Check sheet for the modelled part. Datum: model origin and axes. Units: mm. A direction names the side the tool comes from. Round coordinates to 2 decimals unless told otherwise and drop trailing zeros. Order: outer loops, then holes, each group sorted by start corner. A loop starts at its lowest first (then second) coordinate and runs counter-clockwise, first axis right, second up.
Autodesk Inventor part; units mm, degrees
ref_plane "YZ Plane" through (0, 0, 0) normal (1, 0, 0) x (0, 1, 0)
ref_plane "XZ Plane" through (0, 0, 0) normal (0, 1, 0) x (-1, 0, 0)
ref_plane "XY Plane" through (0, 0, 0) normal (0, 0, 1) x (1, 0, 0)
sketch "Sketch1" plane through (0, 0, 0) normal (0, 0, 1) x (1, 0, 0)
  line L0 (3, 13.65) -> (3, 2.65)
  line L1 (3, 2.65) -> (24, 2.65)
  line L2 (24, 2.65) -> (24, -9)
  line L3 (24, -9) -> (21, -9)
  line L4 (21, -9) -> (21, 0)
  line L5 (21, 0) -> (0, 0)
  line L6 (0, 0) -> (0, 13.65)
  line L7 (0, 13.65) -> (3, 13.65)
  dimension "d0" = 2.65
  dimension "d1" = 21
  dimension "d2" = 9
  dimension "d3" = 3
  dimension "d4" = 3
  dimension "d5" = 11
extrude "Extrusion1" add sketch "Sketch1" along normal blind 45
sketch "Sketch2" plane through (3, 2.65, 0) normal (1, 0, 0) x (0, 0, -1)
  line L0 (0, 11) -> (-45, 11)
  line L1 (-35, 11) -> (-28, 0)
  line L2 (-17, 0) -> (-10, 11)
  line L3 (0, 0) -> (0, 11)
  line L4 (0, 11) -> (-45, 11)
  line L5 (-45, 0) -> (-45, 11)
  line L6 (0, 0) -> (-45, 0)
  point P0 (0, -2.65)
  dimension "d10" = 10
  dimension "d11" = 10
  dimension "d38" = 11
extrude "Extrusion2" cut sketch "Sketch2" against normal through all contours L2 L6 L1 L0
ref_plane "Work Plane1" through (0, 0, 22.5) normal (0, 0, 1) x (1, 0, 0)
sketch "Sketch3" plane through (3, 2.65, 0) normal (0, 1, 0) x (1, 0, 0)
  line L0 (-3, 0) -> (18, 0)
  line L1 (6, 0) -> (9, -3)
  line L2 (9, -3) -> (12, -3)
  line L3 (12, -3) -> (15, 0)
  line L4 (6, -45) -> (9, -42)
  line L5 (9, -42) -> (12, -42)
  line L6 (12, -42) -> (15, -45)
  line L7 (21, 0) -> (0, 0)
  line L8 (0, 0) -> (0, -17)
  line L9 (0, -17) -> (-3, -17)
  line L10 (-3, -28) -> (-3, -17)
  line L11 (0, -28) -> (-3, -28)
  line L12 (0, -28) -> (0, -45)
  line L13 (21, -45) -> (0, -45)
  line L14 (21, 0) -> (21, -45)
  point P0 (10.5, -3)
  point P1 (10.5, 0)
  point P2 (10.5, -42)
  point P3 (10.5, -45)
  dimension "d14" = 45
  dimension "d15" = 45
  dimension "d16" = 3
  dimension "d17" = 3
  dimension "d18" = 3
extrude "Extrusion3" cut sketch "Sketch3" against normal through all contours L0 L3 L2 L1 | L13 L4 L5 L6
sketch "Sketch4" plane through (3, 2.65, 45) normal (1, 0, 0) x (0, 0, -1)
  line L0 (0, 0) -> (0, 11)
  line L1 (45, 0) -> (45, 11)
  line L2 (45, 11) -> (35, 11)
  line L3 (10, 11) -> (0, 11)
  point P0 (45, -2.65)
  point P1 (40.5, 5.85)
  point P2 (4.5, 5.85)
  point P3 (0, 5.5)
  point P4 (45, 5.5)
  dimension "d21" = 4.5
  dimension "d22" = 4.5
  dimension "d46" = 5.15
hole "Hole1" at (3, 8.5, 4.5) at (3, 8.5, 40.5) direction (-1, 0, 0) diameter 3.6 end through all countersink diameter 6.3 countersink angle 90
sketch "Sketch5" plane through (21, -9, 0) normal (0, -1, 0) x (1, 0, 0)
  line L0 (0, 0) -> (3, 0)
  line L1 (3, 0) -> (3, 45)
  line L2 (0, 45) -> (3, 45)
  line L3 (0, 0) -> (0, 45)
  line L4 (3, 0) -> (3, 45)
  line L5 (3, 19.1965) -> (11, 13.5983)
  line L6 (11, 13.5983) -> (11, 5.5983)
  line L7 (11, 5.5983) -> (3, 0)
  line L8 (3, 45) -> (11, 39.4017)
  line L9 (11, 39.4017) -> (11, 31.4017)
  line L10 (11, 31.4017) -> (3, 25.8035)
  line L11 (3, 0) -> (-3, 0)
  line L12 (3, 45) -> (-3, 45)
  point P0 (-21, 0)
  point P1 (3, 22.5)
  dimension "d30" = 8
  dimension "d31" = 8
  dimension "d32" = 8
  dimension "d33" = 8
  dimension "d66" = 5.5983
  dimension "d67" = 5.5983
extrude "Extrusion4" add sketch "Sketch5" against normal blind 3 contours L1 L5 L6 L7 | L8 L9 L10 L1
sketch "Sketch6" plane through (21, -6, 0) normal (0, 1, 0) x (1, 0, 0)
  line L0 (3, -19.1965) -> (11, -13.5983)
  line L1 (11, -13.5983) -> (11, -5.5983)
  line L2 (11, -5.5983) -> (3, 0)
  line L3 (3, -19.1965) -> (3, 0)
  line L4 (3, -45) -> (11, -39.4017)
  line L5 (11, -39.4017) -> (11, -31.4017)
  line L6 (11, -31.4017) -> (3, -25.8035)
  line L7 (3, -19.1965) -> (3, 0)
  line L8 (3, -45) -> (3, -25.8035)
  line L9 (3, -19.1965) -> (11, -13.5983)
  line L10 (11, -13.5983) -> (11, -5.5983)
  line L11 (11, -5.5983) -> (3, 0)
  line L12 (3, -45) -> (11, -39.4017)
  line L13 (11, -39.4017) -> (11, -31.4017)
  line L14 (11, -31.4017) -> (3, -25.8035)
  line L15 (3, -45) -> (3, -25.8035)
  point P0 (-21, 0)
  point P1 (6, -35.4017)
  point P2 (6, -9.5983)
  point P3 (7, -16.3974)
  point P4 (7, -28.6026)
  point P5 (11, -35.4017)
  point P6 (11, -9.5983)
  dimension "d62" = 3
hole "Hole2" at (27, -6, 35.4017) at (27, -6, 9.5983) direction (0, -1, 0) diameter 3.6 end through all countersink diameter 6.3 countersink angle 90
sketch "Sketch7" plane through (24, 2.65, 45) normal (0, 1, 0) x (1, 0, 0)
  circle A0 centre (-10.5, 36) radius 2
  circle A1 centre (-10.5, 9) radius 2
  circle A2 centre (-10.5, 9) radius 4
  circle A3 centre (-10.5, 36) radius 4
  line L0 (-12, 3) -> (-9, 3)
  line L1 (-24, 17) -> (-24, 28)
  line L2 (-24, 22.5) -> (-9, 22.5) construction
  point P0 (-24, 45)
  point P1 (-10.5, 3)
  dimension "d48" = 4
  dimension "d49" = 13.5
  dimension "d50" = 13.5
  dimension "d51" = 8
  dimension "d61" = 27
extrude "Extrusion5" add sketch "Sketch7" along normal blind 3
extrude "Extrusion6" cut sketch "Sketch7" against normal through all contours A0 | A1
draft "FaceDraft1" angle 30 pull direction (0, 1, 0) faces at (17.487, 4.65, 36.3219) fixed edges at (9.5, 5.65, 36)
draft "FaceDraft2" angle 30 pull direction (0, 1, 0) faces at (17.487, 4.65, 9.3219) fixed edges at (9.5, 5.65, 9)
equation "\"d30\" = d31"
equation "\"d32\" = d31"
equation "\"d33\" = d30"
equation "\"d50\" = d49"
properties part number "ESC Mount"
Item 1: Access from +Z, -Z, +X, -X, +Y, -Y to the whole of each face (thin tool, end or side, straight path). Record for faces 5 (the cylindrical face through (12.026, 2.865, 7.648)), 6 (the flat face through (16, 1, 2)), 7 (the flat face through (30, -6, 8)), 8 (the flat face through (11, 0, 22)), 9 (the flat face through (28.056, -7.521, 28.642)).
Answer:
face 5: +Y, -Y
face 6: -Z, +Y, -Y
face 7: +Z, -Z, +X, +Y
face 8: +Z, -Z, -X, -Y
face 9: +X, +Y, -Y
Item 2: Release check for a two-part mould opening along Z. For faces 1 (the flat face through (1, 13.65, 40)), 2 (the flat face through (22, -2, 0)), 3 (the flat face through (27.94, -7.52, 16.44)), 4 (the flat face through (10, 1, 44)) record: released by +Z, released by -Z, zero draft, split by the parting line, or undercut.
Answer:
face 1: zero draft
face 2: released by -Z
face 3: undercut
face 4: released by +Z
Item 3: Sectioned sample at D-D (x = 27). Record the cut outline in (y, z).
Answer:
outline: (-9, 2.1) - (-6, 2.1) - (-6, 6.45) - (-7.35, 7.8) - (-9, 7.8) - close; (-9, 11.4) - (-7.35, 11.4) - (-6, 12.75) - (-6, 17.1) - (-9, 17.1) - close; (-9, 27.9) - (-6, 27.9) - (-6, 32.25) - (-7.35, 33.6) - (-9, 33.6) - close; (-9, 37.2) - (-7.35, 37.2) - (-6, 38.55) - (-6, 42.9) - (-9, 42.9) - close
Item 4: Sectioned sample at C-C (y = 8.5). Record the cut outline in (x, z).
Answer:
outline: (0, 0) - (3, 0) - (3, 1.35) - (1.65, 2.7) - (0, 2.7) - close; (0, 6.3) - (1.65, 6.3) - (3, 7.65) - (3, 13.28) - (0, 13.28) - close; (0, 31.72) - (3, 31.72) - (3, 37.35) - (1.65, 38.7) - (0, 38.7) - close; (0, 42.3) - (1.65, 42.3) - (3, 43.65) - (3, 45) - (0, 45) - close
Item 5: Scan lines: line 1 along Z through (x, y) = (13.5, 1.8); line 2 along Z through (x, y) = (27, -7.7); line 3 along Z through (x, y) = (0.65, 8.5). Record each from-to range of solid material in increasing order.
Answer:
line 1: z = 3 to 7, 11 to 34, 38 to 42
line 2: z = 2.1 to 7.8, 11.4 to 17.1, 27.9 to 33.6, 37.2 to 42.9
line 3: z = 0 to 2.7, 6.3 to 13.28, 31.72 to 38.7, 42.3 to 45
Item 6: Go/stop test with flat-tipped pins: P1, Ø9, axis at x = 29, z = 30.5, coming from the +Y side; P2, Ø8, axis at y = 10, z = 17, coming from the -X side; P3, Ø4, axis at x = 12, z = 35.5, coming from the +Y side; P4, Ø12, axis at y = 10.5, z = 9.5, coming from the +X side. Record where each tip stops, or that it passes through.
Answer:
P1: stops at y = -6
P2: stops at x = 0
P3: stops at y = 5.65
P4: stops at x = 18.16
Item 7: Sectioned sample at A-A (x = 13.5). Record the cut outline in (y, z).
Answer:
outline: (0, 3) - (2.65, 3) - (2.65, 3.27) - (5.65, 5) - (5.65, 7) - (0, 7) - close; (0, 11) - (5.65, 11) - (5.65, 13) - (2.65, 14.73) - (2.65, 30.27) - (5.65, 32) - (5.65, 34) - (0, 34) - close; (0, 38) - (5.65, 38) - (5.65, 40) - (2.65, 41.73) - (2.65, 42) - (0, 42) - close
Item 8: Sectioned sample at B-B (z = 24). Record the cut outline in (x, y), and give its area (3 significant figures).
Answer:
outline: (0, 0) - (21, 0) - (21, -9) - (24, -9) - (24, 2.65) - (0, 2.65) - close
area: 90.6 mm2
